```python
from build123d import *

# Parameters (mm, degrees)
SKETCH1_W           = 35
SKETCH1_H           = 35
BOSS_EXTRUDE1_DEPTH = 19
SKETCH2_W           = 35
SKETCH2_H           = 14
BOSS_EXTRUDE2_DEPTH = 35
SKETCH3_R           = 3
CUT_EXTRUDE1_DEPTH  = 68.690472003
SKETCH4_R           = 9
CUT_EXTRUDE2_DEPTH  = 2
SKETCH6_R           = 1.5
CUT_EXTRUDE3_DEPTH  = 68.690472003
SKETCH7_R           = 1.7
CUT_EXTRUDE4_DEPTH  = 61.621778265


with BuildPart() as part:
    # Sketch1 → Boss-Extrude1 (new body)
    with BuildSketch(Plane.XY):
        with Locations((17.5, 17.5)):
            Rectangle(SKETCH1_W, SKETCH1_H)
    extrude(amount=BOSS_EXTRUDE1_DEPTH)

    # Sketch2 → Boss-Extrude2 (add)
    with BuildSketch(Plane.XY.offset(19)):
        with Locations((17.5, 7)):
            Rectangle(SKETCH2_W, SKETCH2_H)
    extrude(amount=BOSS_EXTRUDE2_DEPTH)

    # Sketch3 → Cut-Extrude1 (cut, through all)
    with BuildSketch(Plane(origin=(0, 14, 0), x_dir=(1, 0, 0), z_dir=(0, 1, 0))):
        with Locations(Location((17.5, -36.5, 0), (0, 0, 270))):
            Circle(SKETCH3_R)
    extrude(amount=-CUT_EXTRUDE1_DEPTH, mode=Mode.SUBTRACT)

    # Sketch4 → Cut-Extrude2 (cut)
    with BuildSketch(Plane(origin=(0, 14, 0), x_dir=(1, 0, 0), z_dir=(0, 1, 0))):
        with Locations(Location((17.5, -36.5, 0), (0, 0, 270))):
            Circle(SKETCH4_R)
    extrude(amount=-CUT_EXTRUDE2_DEPTH, mode=Mode.SUBTRACT)

    # Sketch6 → Cut-Extrude3 (cut, through all)
    with BuildSketch(Plane(origin=(0, 14, 0), x_dir=(1, 0, 0), z_dir=(0, 1, 0))):
        with Locations(Location((6.5, -36.5, 0), (0, 0, 270))):
            Circle(SKETCH6_R)
        with Locations(Location((17.5, -25.5, 0), (0, 0, 270))):
            Circle(SKETCH6_R)
        with Locations(Location((28.5, -36.5, 0), (0, 0, 270))):
            Circle(SKETCH6_R)
        with Locations(Location((17.5, -47.5, 0), (0, 0, 270))):
            Circle(SKETCH6_R)
    extrude(amount=-CUT_EXTRUDE3_DEPTH, mode=Mode.SUBTRACT)

    # Sketch7 → Cut-Extrude4 (cut, through all)
    with BuildSketch(Plane.XY.offset(19)):
        with Locations((8.75, 29.75)):
            Circle(SKETCH7_R)
        with Locations((26.25, 29.75)):
            Circle(SKETCH7_R)
        with Locations((8.75, 19.25)):
            Circle(SKETCH7_R)
        with Locations((26.25, 19.25)):
            Circle(SKETCH7_R)
    extrude(amount=-CUT_EXTRUDE4_DEPTH, mode=Mode.SUBTRACT)


solid = part.part
```
Work out the finished part from the listing and answer in its coordinate system (mm). A direction names the side the tool comes from. Give positions to 0.01 mm unless a question says otherwise; leave off trailing zeros. Loops run counter-clockwise (first coordinate to the right, second up) from the corner with the lowest first, then second, coordinate; pieces in that order, holes last. Notation, with made-up numbers: (-22.75, -24) -> (27.25, -24) arc R25 cw to (27.25, 12) -> close; hole circle Ø6 at (-30, 68.25). An arc over 180 degrees is marked (long way). Write item = value, one per line. Start each with the question number.
(1) Find section D-D on z = 25.5. Give the vertices of the cut face in (x, y).
(2) Find section C-C on z = 16.5. Give the vertices of the cut face in (x, y).
(3) Find section B-B on x = 17.5. Give the vertices of the cut face in (y, z).
(4) The mould has two halves that part along X. Classify faces 4 (the flat face through (35, 13, 21)), 5 (the cylindrical face through (8.529, 20.936, 9.633)), 6 (the flat face through (17, 7, 54)): +X half, -X half, draft (parallel to the pull), parting line (faces both ways), or undercut.
(5) Which of the six approach directions +Z, -Z, +X, -X, +Y, -Y give full straight-line access (tool end or side, diameter ignored) to faces 1 (the flat face through (9, 14, 32)), 2 (the cylindrical face through (17.57, 7.1, 46)), 3 (the cylindrical face through (17.9, 13.01, 27.51))?
(6) Find section A-A on y = 19.25. Give the vertices of the cut face in (x, z), and give its area (3 significant figures).
(7) Find the intervals of material crossed by probe 1 along Y at (x, z) = (26.25, 7.5); probe 2 along X at (y, z) = (8.5, 36.5); probe 3 along X at (y, z) = (10.5, 25.5), in increasing order. Write a range as from..to.
(8) Given pin 1 Ø17.5 at (x, z) = (25, 31.5) entering from +Y; pin 2 Ø10 at (x, y) = (17.5, 19.5) entering from +Z; pin 3 Ø1 at (x, z) = (12.5, 36.5) entering from +Y, each flat-ended and moving along its own axis, determine where each tip first touches the part or whether it passes through.
From the geometry:
q1.outline = (0, 0) -> (16, 0) -> (16, 14) -> (0, 14) -> close; (19, 0) -> (35, 0) -> (35, 14) -> (19, 14) -> close
q2.outline = (0, 0) -> (35, 0) -> (35, 35) -> (0, 35) -> close; hole circle Ø3.4 at (8.75, 19.25); hole circle Ø3.4 at (8.75, 29.75); hole circle Ø3.4 at (26.25, 19.25); hole circle Ø3.4 at (26.25, 29.75)
q3.outline = (0, 0) -> (35, 0) -> (35, 19) -> (14, 19) -> (14, 24) -> (0, 24) -> close; (0, 27) -> (14, 27) -> (14, 27.5) -> (12, 27.5) -> (12, 33.5) -> (0, 33.5) -> close; (0, 39.5) -> (12, 39.5) -> (12, 45.5) -> (14, 45.5) -> (14, 46) -> (0, 46) -> close; (0, 49) -> (14, 49) -> (14, 54) -> (0, 54) -> close
q4.face_4 = +X half
q4.face_5 = undercut
q4.face_6 = draft
q5.face_1 = +Z, +X, -X, +Y
q5.face_2 = +Y, -Y
q5.face_3 = +Y
q6.outline = (0, 0) -> (7.05, 0) -> (7.05, 19) -> (0, 19) -> close; (10.45, 0) -> (24.55, 0) -> (24.55, 19) -> (10.45, 19) -> close; (27.95, 0) -> (35, 0) -> (35, 19) -> (27.95, 19) -> close
q6.area = 536 mm^2
q7.probe_1 = 0..17.55, 20.95..28.05, 31.45..35
q7.probe_2 = 0..5, 8..14.5, 20.5..27, 30..35
q7.probe_3 = 0..16, 19..35
q8.pin_1 = 14
q8.pin_2 = 19
q8.pin_3 = 12
